Could you check a few things on this model? Use its own coordinates, in mm. A direction names the side the tool comes from. Coordinates: 2 decimals unless noted, no trailing zeros. Loops run counter-clockwise (first coordinate to the right, second up) from the corner with the lowest first, then second, coordinate; pieces in that order, holes last. Notation, with made-up numbers: (-29.75, 82) - (24.25, 82) arc R28 cw to (24.25, 100) - close; hole circle Ø3 at (21.5, -9.75). An arc over 180 degrees is marked (long way). Put each result on its own line as item: value. Start each with the question number.
```python
from build123d import *

# Parameters (mm, degrees)
F0_W     = 390
F0_H     = 900
F1_DEPTH = 780
F2_W     = 800
F2_H     = 400
F3_DEPTH = 20
F4_W     = 750
F4_H     = 850
F4_W_2   = 740
F4_H_2   = 205
F4_R     = 30
F5_DEPTH = 20
F6_W     = 740
F6_H     = 350
F6_W_2   = 700
F6_H_2   = 310
F7_DEPTH = 40
F8_R     = 14.142136
F9_DEPTH = 200


with BuildPart() as f1:
    # F0 (on Right) → F1 (new body)
    with BuildSketch(Plane.YZ):
        with Locations((195, 450)):
            Rectangle(F0_W, F0_H)
    extrude(amount=F1_DEPTH)

    # F2 (on face) → F3 (join)
    with BuildSketch(Plane.XY.offset(900)):
        with Locations((390, 190)):
            Rectangle(F2_W, F2_H)
    extrude(amount=-F3_DEPTH)

    # F4 (on face) → F5 (cut)
    with BuildSketch(Plane.XZ):
        with Locations((390, 440)):
            Rectangle(F4_W, F4_H)
        with Locations((390, 127.5)):
            Rectangle(F4_W_2, F4_H_2, mode=Mode.SUBTRACT)
        with Locations((390, 337.5)):
            Rectangle(F4_W_2, F4_H_2, mode=Mode.SUBTRACT)
        with Locations((390, 547.5)):
            Rectangle(F4_W_2, F4_H_2, mode=Mode.SUBTRACT)
        with Locations((390, 757.5)):
            Rectangle(F4_W_2, F4_H_2, mode=Mode.SUBTRACT)
        with Locations((280, 757.5)):
            Circle(F4_R)
        with Locations((500, 757.5)):
            Circle(F4_R)
        with Locations((280, 547.5)):
            Circle(F4_R)
        with Locations((500, 547.5)):
            Circle(F4_R)
        with Locations((280, 337.5)):
            Circle(F4_R)
        with Locations((500, 337.5)):
            Circle(F4_R)
        with Locations((280, 127.5)):
            Circle(F4_R)
        with Locations((500, 127.5)):
            Circle(F4_R)
    extrude(amount=-F5_DEPTH, mode=Mode.SUBTRACT)

    # F6 (on face) → F7 (join)
    with BuildSketch(Plane(origin=(0, 0, 0), x_dir=(1, 0, 0), z_dir=(0, 0, -1))):
        with Locations((390, -195)):
            Rectangle(F6_W, F6_H)
        with Locations((390, -195)):
            Rectangle(F6_W_2, F6_H_2, mode=Mode.SUBTRACT)
    extrude(amount=F7_DEPTH)

    # F8 (on face) → F9 (join)
    with BuildSketch(Plane(origin=(0, 0, 0), x_dir=(1, 0, 0), z_dir=(0, 0, -1))):
        with Locations((30, -30)):
            Circle(F8_R)
        with Locations((750, -30)):
            Circle(F8_R)
        with Locations((30, -360)):
            Circle(F8_R)
        with Locations((750, -360)):
            Circle(F8_R)
    extrude(amount=F9_DEPTH)


solid = f1.part
```
(1) For pin 1 Ø22 at (y, z) = (9, 386) entering from -X; pin 2 Ø1 at (x, y) = (476, 156) entering from -Z; pin 3 Ø1.5 at (x, z) = (202, 43.5) entering from -Y, each with a flat end and sliding along its axis, tell me the tip position at first contact or that it passes through.
(2) I need wall thicknesses on L1, parallel to X at y = 275, z = -27; L2, parallel to X at y = 225, z = 169; L3, parallel to Y at x = 744.5, z = 641. Which ranges of each line are inside material? Lowest first, please. Write a range as [from, to].
(3) Which directions (+Z, -Z, +X, -X, +Y, -Y) give clear straight access to the entire face, cutting with the end or side of a thin tool? Please do faces 4 (the flat face through (760, 197, -20)), 5 (the cylindrical face through (527.712, 9.86, 326.01)), 6 (the cylindrical face through (763.064, 365.417, -98.6)).
(4) I want a section at D-D on z = 337.5. List the corners of the cut face in (x, y) for me, and give its area (3 significant figures).
(5) I want a section at C-C on y = 266. List the corners of the cut face in (x, z) for me.
(6) I want a section at B-B on z = 72. List the corners of the cut face in (x, y) for me, and give its area (3 significant figures).
(7) If we mould it in two halves opening along Z, with no side actions, what happens to faces 1 (the cylindrical face through (273.497, 9.86, 98.213)), 2 (the flat face through (750, 360, -200)), 3 (the flat face through (13, 0, 242))? For each: pulls with the +Z half, pulls with the -Z half, needs draft (parallel to the pull), parting line crosses it, or undercut.
Answer sheet:
1. pin 1: stops at x = 0
1. pin 2: stops at z = 0
1. pin 3: stops at y = 0
2. L1: x = [20, 40], [740, 760]
2. L2: x = [0, 780]
2. L3: y = [0, 390]
3. face 4: -Z, +X
3. face 5: -Y
3. face 6: -Z
4. outline: (0, 0) - (15, 0) - (15, 20) - (20, 20) - (20, 0) - (250, 0) - (250, 20) - (310, 20) - (310, 0) - (470, 0) - (470, 20) - (530, 20) - (530, 0) - (760, 0) - (760, 20) - (765, 20) - (765, 0) - (780, 0) - (780, 390) - (0, 390) - close
4. area: 302,000 mm^2
5. outline: (-10, 880) - (0, 880) - (0, 0) - (20, 0) - (20, -40) - (40, -40) - (40, 0) - (740, 0) - (740, -40) - (760, -40) - (760, 0) - (780, 0) - (780, 880) - (790, 880) - (790, 900) - (-10, 900) - close
6. outline: (0, 0) - (15, 0) - (15, 20) - (20, 20) - (20, 0) - (760, 0) - (760, 20) - (765, 20) - (765, 0) - (780, 0) - (780, 390) - (0, 390) - close
6. area: 304,000 mm^2
7. face 1: undercut
7. face 2: pulls with the -Z half
7. face 3: needs draft
